For this review, use the dimensioned drawing (mm, ordinates from the lowest corner) and the shaded views. Give positions to 0.01 mm unless a question says otherwise; leave off trailing zeros. Loops run counter-clockwise (first coordinate to the right, second up) from the corner with the lowest first, then second, coordinate; pieces in that order, holes last. Notation, with made-up numbers: (23.25, 42) - (49.25, 42) arc R24 cw to (49.25, 76) - close; hole circle Ø7 at (77.25, 89). An arc over 180 degrees is marked (long way). Write each question's results on one line, items separated by ' | '.
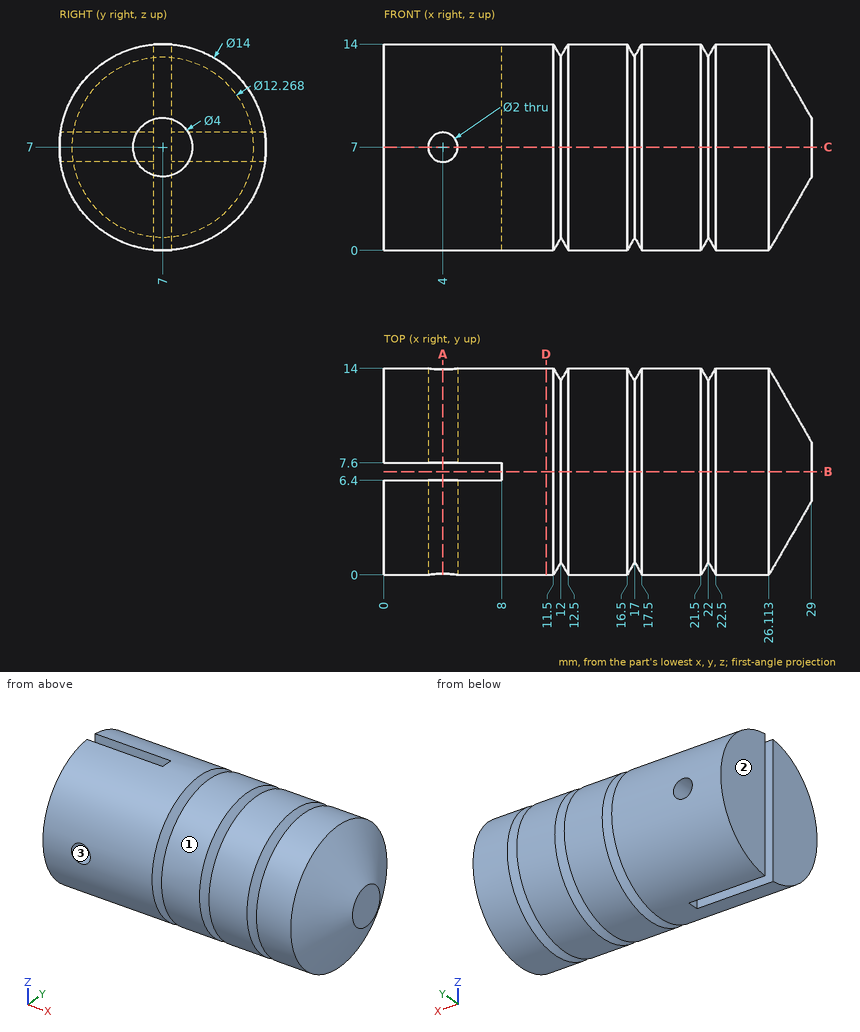
Item 1: We need section A-A on x = 4. Give the boundary of the cut face in (y, z).
Output values:
outline: (0.07, 6) arc R7 ccw to (6.4, 0.03) - (6.4, 6) - close; (0.07, 8) - (6.4, 8) - (6.4, 13.97) arc R7 ccw to start; (7.6, 0.03) arc R7 ccw to (13.93, 6) - (7.6, 6) - close; (7.6, 8) - (13.93, 8) arc R7 ccw to (7.6, 13.97) - close
Item 2: We need section B-B on y = 7. Give the boundary of the cut face in (x, z).
Output values:
outline: (8, 0) - (11.5, 0) - (12, 0.87) - (12.5, 0) - (16.5, 0) - (17, 0.87) - (17.5, 0) - (21.5, 0) - (22, 0.87) - (22.5, 0) - (26.11, 0) - (29, 5) - (29, 9) - (26.11, 14) - (22.5, 14) - (22, 13.13) - (21.5, 14) - (17.5, 14) - (17, 13.13) - (16.5, 14) - (12.5, 14) - (12, 13.13) - (11.5, 14) - (8, 14) - close
Item 3: Clearance check with flat-ended pins moving along their axes: P1, Ø1.8, axis at x = 4, z = 7, coming from the +Y side; P2, Ø3, axis at x = 11, y = 4, coming from the +Z side; P3, Ø1, axis at x = 21, z = 6, coming from the -Y side; P4, Ø3, axis at y = 9.5, z = 11.5, coming from the +X side. State where each tip first meets the part, or that it passes through.
Output values:
P1: passes through | P2: stops at z = 13.84 | P3: stops at y = 0.02 | P4: stops at x = 28.05
Item 4: Wall thickness on probe 1 along X at (y, z) = (11.5, 11.5); probe 2 along Y at (x, z) = (7, 7.25); probe 3 along X at (y, z) = (11.25, 1.5): over which ranges is each line inside the solid? List them lowest first.
Output values:
probe 1: x = 0 to 11.87, 12.13 to 16.87, 17.13 to 21.87, 22.13 to 26.48 | probe 2: y = 0 to 6.4, 7.6 to 14 | probe 3: x = 0 to 11.53, 12.47 to 16.53, 17.47 to 21.53, 22.47 to 26.14
Item 5: We need section C-C on z = 7. Give the number of separate pieces and of enclosed holes in the cut face, then the cut area to 3 significant figures.
Output values:
separate pieces: 3 | enclosed holes: 0 | area: 354 mm²
Item 6: We need section D-D on x = 11. Give the boundary of the cut face in (y, z), then the cut area to 3 significant figures.
Output values:
outline: circle Ø14 at (7, 7) | area: 154 mm²
Item 7: Draft analysis for pull direction Z (two halves, no side actions). For the marked faces 1, 2 and 3, state which applies: +Z half, -Z half, draft (parallel to the pull), parting line (faces both ways), or undercut.
Output values:
face 1: parting line | face 2: draft | face 3: undercut
